Can you work these out from the model? Positions are in its coordinate system, mm. Round coordinates to 2 decimals unless told otherwise and drop trailing zeros. Order: outer loops, then holes, each group sorted by start corner. A loop starts at its lowest first (then second) coordinate and runs counter-clockwise, first axis right, second up. Notation, with made-up numbers: (74.25, -14.75) -> (125.25, -14.75) arc R11 ccw to (125.25, 4.25) -> close; hole circle Ø6 at (-37.75, -34). An arc over 180 degrees is marked (long way). One line per item, written item: value.
```python
from build123d import *

# Parameters (mm, degrees)
F0_W     = 50
F0_H     = 140
F1_DEPTH = 3
F4_D     = 5


with BuildPart() as f1:
    # F0 (on Top) → F1 (new body)
    with BuildSketch(Plane.XY):
        with Locations((25, 70)):
            Rectangle(F0_W, F0_H)
    extrude(amount=F1_DEPTH)

    # F4 (through all)
    with Locations(Plane.XY.offset(3)):
        with Locations((40, 75), (40, 25)):
            Hole(F4_D / 2)


solid = f1.part
```
Q1. I want a section at A-A on x = 40. List the corners of the cut face in (y, z) for me.
Answers below:
outline: (0, 0) -> (22.5, 0) -> (22.5, 3) -> (0, 3) -> close; (27.5, 0) -> (72.5, 0) -> (72.5, 3) -> (27.5, 3) -> close; (77.5, 0) -> (140, 0) -> (140, 3) -> (77.5, 3) -> close
Q2. We'd pull the mould along X, two halves only. Please class faces 1 (the face through (37.69, 74.04, 1.48)), 2 (the face through (38.66, 27.11, 1.48)), 3 (the face through (0, 69, 1)), 4 (the face through (25, 0, 1)): released by +X, released by -X, zero draft, split by the parting line, or undercut.
Answers below:
face 1: undercut
face 2: undercut
face 3: released by -X
face 4: zero draft
Q3. Please list where these lines run through material, in increasing order: line 1 along Y through (x, z) = (40, 0.85); line 2 along Y through (x, z) = (38.5, 1.5).
Answers below:
line 1: 0 to 22.5, 27.5 to 72.5, 77.5 to 140
line 2: 0 to 23, 27 to 73, 77 to 140
Q4. I want a section at B-B on y = 75. List the corners of the cut face in (x, z) for me, plus the area to 3 significant figures.
Answers below:
outline: (0, 0) -> (37.5, 0) -> (37.5, 3) -> (0, 3) -> close; (42.5, 0) -> (50, 0) -> (50, 3) -> (42.5, 3) -> close
area: 135 mm^2
